Could you check a few things on this drawing? It's one solid part, dimensions in mm from its lowest x, y, z. A direction names the side the tool comes from. Coordinates: 2 decimals unless noted, no trailing zeros. Write each loop counter-clockwise with the first axis right and the second up, starting at its lowest first coordinate (ties: lowest second). Pieces come first, ordered by that corner, then holes.
Item 1: Please list where these lines run through material, in increasing order: line 1 (Z direction, x = 13.75, y = 6.25); line 2 (Z direction, x = 6, y = 3); line 3 (Z direction, x = 5, y = 22.75).
Item 2: If we mould it in two halves opening along Z, with no side actions, what happens to the marked faces 1, 2, 3 and 4? For each: pulls with the +Z half, pulls with the -Z half, needs draft (parallel to the pull), parting line crosses it, or undercut.
Item 3: I'm going to push flat-ended pins straight in: P1, Ø5, axis at y = 16, z = 24.5, coming from the -X side; P2, Ø1, axis at y = 16, z = 71.5, coming from the -X side; P3, Ø3, axis at x = 5.5, z = 133, coming from the +Y side. Where does each tip first touch, or does it pass through?
Item 4: I want a section at A-A (z = 27). Please give me the cut outline in (x, y).
Item 5: For the marked faces 5, 6, 7, 8 and 9, which set-ups out of +Z, -Z, +X, -X, +Y, -Y let a thin tool reach every point of the face, with its end or its side?
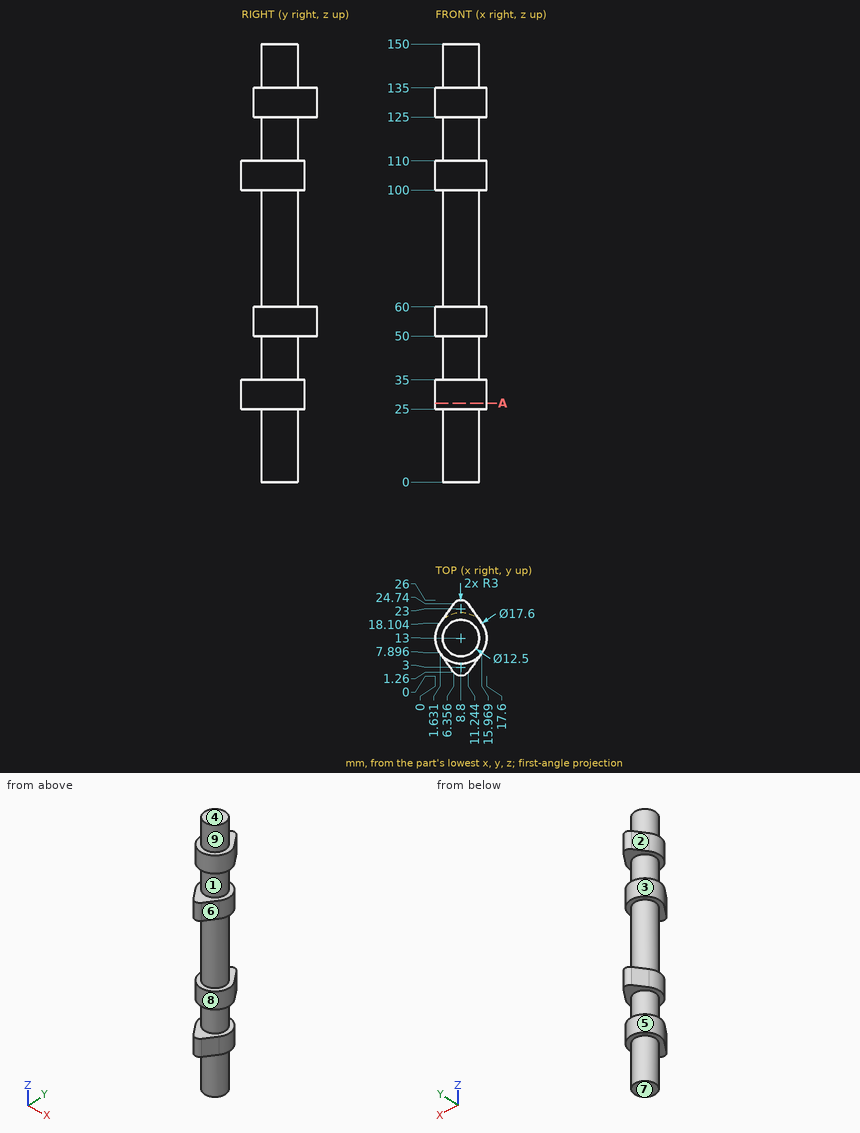
Answer:
1. line 1: z = 25 to 35, 50 to 60, 100 to 110, 125 to 135
1. line 2: z = 25 to 35, 100 to 110
1. line 3: z = 50 to 60, 125 to 135
2. face 1: undercut
2. face 2: needs draft
2. face 3: undercut
2. face 4: pulls with the +Z half
3. P1: stops at x = 0.02
3. P2: stops at x = 3.07
3. P3: stops at y = 25.4
4. outline: (1.63, 7.9) - (6.36, 1.26) arc R3 ccw to (11.24, 1.26) - (15.97, 7.9) arc R8.8 ccw (long way) to start
5. face 5: -Z
5. face 6: +Z, -Z, +X, -Y
5. face 7: -Z, +X, -X, +Y, -Y
5. face 8: none
5. face 9: +Z
